from build123d import *

# Parameters (mm, degrees)
BOSS_EXTRUDE1_DEPTH = 10.16
BOSS_EXTRUDE2_DEPTH = 10.16
CHAMFER1_SIZE       = 2.54


with BuildPart() as part:
    # Sketch3 → Boss-Extrude1 (new body)
    with BuildSketch(Plane(origin=(0, 0, 0), x_dir=(0, 0, -1), z_dir=(1, 0, 0))):
        Polygon((-101.845577666, -9.102652747), (-95.495577666, -9.102652747), (-95.495577666, 9.947347253), (-89.145577666, 9.947347253), (-89.145577666, 22.647347253), (-51.045577666, 22.647347253), (-51.045577666, 9.947347253), (-44.695577666, 9.947347253), (-44.695577666, -9.102652747), (-38.345577666, -9.102652747), (-38.345577666, 28.997347253), (-101.845577666, 28.997347253), align=None)
    extrude(amount=BOSS_EXTRUDE1_DEPTH)

    # Sketch4 → Boss-Extrude2 (add)
    with BuildSketch(Plane(origin=(10.16, 0, 0), x_dir=(0, 0, -1), z_dir=(1, 0, 0))):
        with BuildLine():
            Line((-101.845577666, -4.773598811), (-101.845577666, 6.888293317))
            ThreePointArc((-101.845577666, 6.888293317), (-93.971577666, 1.057347253), (-101.845577666, -4.773598811))
        make_face()
        with BuildLine():
            Line((-38.345577666, -4.773598811), (-38.345577666, 6.888293317))
            ThreePointArc((-38.345577666, 6.888293317), (-46.219577666, 1.057347253), (-38.345577666, -4.773598811))
        make_face()
    extrude(amount=-BOSS_EXTRUDE2_DEPTH)

    # Chamfer1
    chamfer1_edges = [part.edges().sort_by_distance(p)[0] for p in [
        (5.08, 9.947347253, 44.695577666),
        (5.08, 9.947347253, 95.495577666),
    ]]
    chamfer(chamfer1_edges, length=CHAMFER1_SIZE)


solid = part.part
Can you work these out from the model? Positions are in its coordinate system, mm. A direction names the side the tool comes from. Coordinates: 2 decimals unless noted, no trailing zeros. Write each loop counter-clockwise with the first axis right and the second up, starting at its lowest first coordinate (ties: lowest second). Pieces come first, ordered by that corner, then holes. Notation, with made-up numbers: M 8.25,86 L 52.25,86 A23 cw 52.25,119 Z; hole C 80.5,77.25 d2. An arc over 180 degrees is marked long. Use one line per item in the form item = value.
Q1. If we section it at A-A (y = 12.5): Write out the boundary of the cut face in (x, z), then the cut area to 3 significant figures.
Model answer:
outline = M 0,38.35 L 10.16,38.35 L 10.16,51.05 L 0,51.05 Z; M 0,89.15 L 10.16,89.15 L 10.16,101.85 L 0,101.85 Z
area = 258 mm^2
Q2. I need wall thicknesses on line 1 along Z through (x, y) = (7, 14); line 2 along Y through (x, z) = (8, 83.5); line 3 along Y through (x, z) = (6.5, 49). Which ranges of each line are inside material? Lowest first, please. Write a range as from..to.
Model answer:
line_1 = 38.35..51.05, 89.15..101.85
line_2 = 22.65..29
line_3 = 9.95..29
Q3. For P1, Ø5, axis at x = 6.5, z = 70, coming from the -Y side; P2, Ø2, axis at x = 9, z = 92.5, coming from the -Y side; P3, Ø3, axis at x = 3.5, z = 50, coming from the -Y side, each with a flat end and sliding along its axis, tell me the tip position at first contact or that it passes through.
Model answer:
P1 = 22.65
P2 = 9.4
P3 = 9.95
Q4. If we section it at D-D (z = 91): Write out the boundary of the cut face in (x, y).
Model answer:
outline = M 0,9.95 L 10.16,9.95 L 10.16,29 L 0,29 Z
Q5. If we section it at C-C (z = 70.5): Write out the boundary of the cut face in (x, y), then the cut area to 3 significant figures.
Model answer:
outline = M 0,22.65 L 10.16,22.65 L 10.16,29 L 0,29 Z
area = 64.5 mm^2
Q6. We'd pull the mould along Z, two halves only. Please class faces 1 (the flat face through (5, -9.103, 42)), 2 (the flat face through (5, 9.947, 49)), 3 (the flat face through (5, 10, 101.846)): +Z half, -Z half, draft (parallel to the pull), parting line (faces both ways), or undercut.
Model answer:
face_1 = draft
face_2 = undercut
face_3 = +Z half
Q7. If we section it at B-B (x = 7): Write out the boundary of the cut face in (y, z).
Model answer:
outline = M -9.1,38.35 L 29,38.35 L 29,101.85 L -9.1,101.85 L -9.1,95.5 L -2.97,95.5 A6.1 ccw 5.09,95.5 L 7.41,95.5 L 9.95,92.96 L 9.95,89.15 L 22.65,89.15 L 22.65,51.05 L 9.95,51.05 L 9.95,47.24 L 7.41,44.7 L 5.09,44.7 A6.1 ccw -2.97,44.7 L -9.1,44.7 Z
Q8. For faces 4 (the flat face through (5, 16, 51.046)), 5 (the flat face through (10.16, 23, 71)), 6 (the cylindrical face through (5.15, 1.12, 93.97)), which set-ups out of +Z, -Z, +X, -X, +Y, -Y let a thin tool reach every point of the face, with its end or its side?
Model answer:
face_4 = +X, -X, -Y
face_5 = +Z, -Z, +X, +Y, -Y
face_6 = +X, -X
